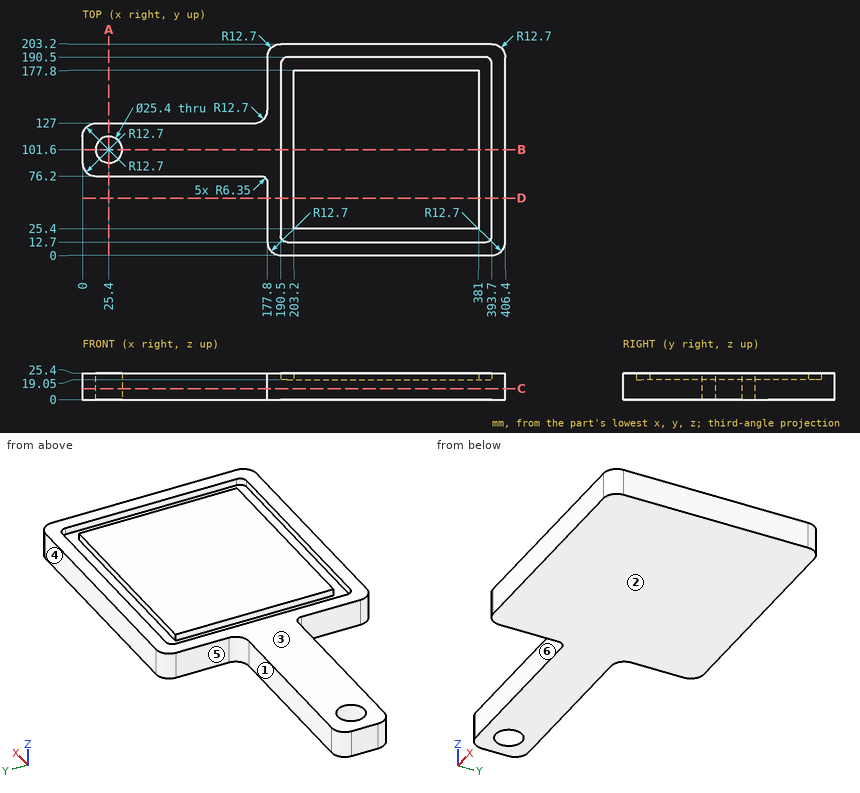
Geometry: see drawing. Coordinates: mm, zero at the bounding-box minimum. A direction names the side the tool comes from. Give positions to 0.01 mm unless a question says otherwise; leave off trailing zeros. Order: outer loops, then holes, each group sorted by start corner. A loop starts at its lowest first (then second) coordinate and runs counter-clockwise, first axis right, second up. Notation, with made-up numbers: M 81.5,19.25 L 107.5,19.25 A20 cw 107.5,24.25 Z; hole C 5.5,66.25 d2. An arc over 180 degrees is marked long. Answer as a JSON object with one key per item and string values.
1. Pull-direction query (Z, two-part tool) for the marked faces 1, 2 and 3; classes: +Z half, -Z half, draft (parallel to the pull), parting line (faces both ways), or undercut.
Result sheet:
{"face 1": "draft", "face 2": "-Z half", "face 3": "+Z half"}
2. Cut plane C-C, the plane z = 10.75. Output: boundary loops of the cut face in (x, y), and give its area (3 significant figures).
Result sheet:
{"outline": "M 0,88.9 A12.7 ccw 12.7,76.2 L 171.45,76.2 A6.35 cw 177.8,69.85 L 177.8,12.7 A12.7 ccw 190.5,0 L 393.7,0 A12.7 ccw 406.4,12.7 L 406.4,190.5 A12.7 ccw 393.7,203.2 L 190.5,203.2 A12.7 ccw 177.8,190.5 L 177.8,139.7 A12.7 cw 165.1,127 L 12.7,127 A12.7 ccw 0,114.3 Z; hole C 25.4,101.6 d25.4", "area": "54,800 mm²"}
3. Ray query, line 1 (Y direction, x = 304, z = 24); line 2 (Y direction, x = 25.4, z = 19.75); line 3 (X direction, y = 73, z = 21.5). Return the intervals inside material, ascending. Write a range as [from, to].
Result sheet:
{"line 1": "[0, 12.7], [25.4, 177.8], [190.5, 203.2]", "line 2": "[76.2, 88.9], [114.3, 127]", "line 3": "[176.96, 190.5], [203.2, 381], [393.7, 406.4]"}
4. First-contact query: P1, Ø7.5, axis at y = 27.5, z = 8.5, coming from the -X side; P2, Ø15, axis at x = 25.4, y = 101.6, coming from the +Z side; P3, Ø5, axis at y = 85, z = 22, coming from the -X side. Flat tips, straight axial feed; report the tip coordinate or a pass-through.
Result sheet:
{"P1": "x = 177.8", "P2": "through", "P3": "x = 0.08"}
5. Reachability of the marked faces 4, 5 and 6 from +Z, -Z, +X, -X, +Y, -Y: full face, straight path, thin tool, end or side. Return the list, or none.
Result sheet:
{"face 4": "+Z, -Z, +X, -X, +Y", "face 5": "+Z, -Z, -X, +Y", "face 6": "+Z, -Z, -X, -Y"}
6. Cut plane A-A, the plane x = 25.4. Output: boundary loops of the cut face in (y, z), and give its area (3 significant figures).
Result sheet:
{"outline": "M 76.2,0 L 88.9,0 L 88.9,25.4 L 76.2,25.4 Z; M 114.3,0 L 127,0 L 127,25.4 L 114.3,25.4 Z", "area": "645 mm²"}
7. Cut plane D-D, the plane y = 55. Output: boundary loops of the cut face in (x, z).
Result sheet:
{"outline": "M 177.8,0 L 406.4,0 L 406.4,25.4 L 393.7,25.4 L 393.7,19.05 L 381,19.05 L 381,25.4 L 203.2,25.4 L 203.2,19.05 L 190.5,19.05 L 190.5,25.4 L 177.8,25.4 Z"}
8. Cut plane B-B, the plane y = 101.6. Output: boundary loops of the cut face in (x, z), and give its area (3 significant figures).
Result sheet:
{"outline": "M 0,0 L 12.7,0 L 12.7,25.4 L 0,25.4 Z; M 38.1,0 L 406.4,0 L 406.4,25.4 L 393.7,25.4 L 393.7,19.05 L 381,19.05 L 381,25.4 L 203.2,25.4 L 203.2,19.05 L 190.5,19.05 L 190.5,25.4 L 38.1,25.4 Z", "area": "9,520 mm²"}
